Read the model definition and answer for the solid it produces. Units are mm, in the model's axes. A direction names the side the tool comes from. Give positions to 0.01 mm unless a question says otherwise; leave off trailing zeros. Write each loop counter-clockwise with the first axis right and the second up, starting at its lowest first coordinate (ties: lowest second). Pieces come first, ordered by that corner, then holes. Notation, with made-up numbers: (66, 43) - (114, 43) arc R24 ccw to (114, 77) - close; hole circle Ø7 at (58.5, 5). An arc over 180 degrees is marked (long way). Answer as CSV lines item,"result".
```python
from build123d import *

# Parameters (mm, degrees)
F0_W     = 410
F0_H     = 42
F1_DEPTH = 19


with BuildPart() as f1:
    # F0 (on Front) → F1 (new body)
    with BuildSketch(Plane.XZ):
        with Locations((0, 215.529412)):
            Rectangle(F0_W, F0_H)
        Polygon((205, 236.529412), (205, 194.529412), (205, -221.470588), (205, -263.470588), (247, -263.470588), (247, 236.529412), align=None)
        Polygon((-205, -221.470588), (-205, 194.529412), (-205, 236.529412), (-247, 236.529412), (-247, -263.470588), (-205, -263.470588), align=None)
        with Locations((0, -242.470588)):
            Rectangle(F0_W, F0_H)
    extrude(amount=F1_DEPTH)


solid = f1.part
```
(1) Find the intervals of material crossed by L1, parallel to Z at x = -83, y = -13.25; L2, parallel to X at y = -13.5, z = -57, in increasing order.
Worked out:
L1,"z = -263.47 to -221.47, 194.53 to 236.53"
L2,"x = -247 to -205, 205 to 247"
(2) A cutting plane is placed at B-B (y = -9.5). Write down the section's boundary in (x, z), and give its area (3 significant figures).
Worked out:
outline,"(-247, -263.47) - (247, -263.47) - (247, 236.53) - (-247, 236.53) - close; hole (-205, -221.47) - (205, -221.47) - (205, 194.53) - (-205, 194.53) - close"
area,"76,400 mm^2"
(3) For faces 1 (the flat face through (216, -19, -10)), 2 (the flat face through (205, -9, -11)), determine the directions among +Z, -Z, +X, -X, +Y, -Y from which every point of the face is accessible in a straight line to the end or side of a thin tool.
Worked out:
face 1,"+Z, -Z, +X, -X, -Y"
face 2,"+Y, -Y"
(4) A cutting plane is placed at A-A (x = 171.5). Write down the section's boundary in (y, z), and give its area (3 significant figures).
Worked out:
outline,"(-19, -263.47) - (0, -263.47) - (0, -221.47) - (-19, -221.47) - close; (-19, 194.53) - (0, 194.53) - (0, 236.53) - (-19, 236.53) - close"
area,"1,600 mm^2"
(5) The mould has two halves that part along Z. Classify faces 3 (the flat face through (-3, -9, 194.529)), 4 (the flat face through (-205, -9, -16)), 5 (the flat face through (216, 0, -10)), 6 (the flat face through (-3, -9, -263.471)): +Z half, -Z half, draft (parallel to the pull), parting line (faces both ways), or undercut.
Worked out:
face 3,"undercut"
face 4,"undercut"
face 5,"draft"
face 6,"-Z half"
(6) A cutting plane is placed at C-C (z = -105). Write down the section's boundary in (x, y).
Worked out:
outline,"(-247, -19) - (-205, -19) - (-205, 0) - (-247, 0) - close; (205, -19) - (247, -19) - (247, 0) - (205, 0) - close"
